Input: part model. Units: mm. Frame: model coordinates. A direction names the side the tool comes from. Round coordinates to 2 decimals unless told otherwise and drop trailing zeros. Write each loop counter-clockwise with the first axis right and the second up, starting at its lowest first coordinate (ties: lowest second). Pieces come first, ordered by that corner, then holes. Notation, with made-up numbers: (-13.5, -11) -> (-6.5, -11) arc R30 cw to (-6.5, 17) -> close; hole circle Ø10 at (-14.75, -40). An arc over 180 degrees is marked (long way). Write item = value, one per line.
```python
from build123d import *

# Parameters (mm, degrees)
EXTRUDE_1_DEPTH   = 15.1
SKETCH_2_R        = 2.5
EXTRUDE_2_DEPTH   = 1.5
EXTRUDE_3_DEPTH   = 1.5
M1_6X0_35_1_D     = 1.25
M1_6X0_35_1_DEPTH = 4.95
M1_6X0_35_1_TIP   = 0.375537887
EXTRUDE_4_DEPTH   = 14.9
SKETCH_7_3_W      = 1
SKETCH_7_3_H      = 2
EXTRUDE_5_DEPTH   = 12.9
SKETCH_8_R        = 2
EXTRUDE_6_DEPTH   = 1.1
EXTRUDE_7_DEPTH   = 1.5
SKETCH_10_R       = 1.2
SKETCH_10_R_2     = 0.65
EXTRUDE_13_DEPTH  = 25


with BuildPart() as part:
    # Sketch 1 → Extrude 1 (new body)
    with BuildSketch(Plane.XY):
        with BuildLine():
            Line((-40.194845485, 23.273623853), (-32.294845485, 23.273623853))
            ThreePointArc((-32.294845485, 23.273623853), (-30.880631923, 22.687837416), (-30.294845485, 21.273623853))
            Line((-30.294845485, 21.273623853), (-30.294845485, 11.373623853))
            ThreePointArc((-30.294845485, 11.373623853), (-30.880631923, 9.959410291), (-32.294845485, 9.373623853))
            Line((-32.294845485, 9.373623853), (-40.194845485, 9.373623853))
            ThreePointArc((-40.194845485, 9.373623853), (-41.609059048, 9.959410291), (-42.194845485, 11.373623853))
            Line((-42.194845485, 11.373623853), (-42.194845485, 21.273623853))
            ThreePointArc((-42.194845485, 21.273623853), (-41.609059048, 22.687837416), (-40.194845485, 23.273623853))
        make_face()
    extrude(amount=EXTRUDE_1_DEPTH)

    # Sketch 2 → Extrude 2 (add)
    with BuildSketch(Plane.XY.offset(15.1)):
        with Locations((-36.244845485, 16.323623853)):
            Circle(SKETCH_2_R)
    extrude(amount=EXTRUDE_2_DEPTH)

    # Sketch 3 → Extrude 3 (add)
    with BuildSketch(Plane(origin=(0, 23.273623853, 0), x_dir=(1, 0, 0), z_dir=(0, 1, 0))):
        with BuildLine():
            Line((-33.744845485, -10.6), (-38.744845485, -10.6))
            ThreePointArc((-38.744845485, -10.6), (-39.098398876, -10.746446609), (-39.244845485, -11.1))
            Line((-39.244845485, -11.1), (-39.244845485, -15.1))
            Line((-39.244845485, -15.1), (-38.744845485, -15.1))
            Line((-38.744845485, -15.1), (-38.744845485, -14.6))
            Line((-38.744845485, -14.6), (-38.744845485, -11.6))
            ThreePointArc((-38.744845485, -11.6), (-38.598398876, -11.246446609), (-38.244845485, -11.1))
            Line((-38.244845485, -11.1), (-34.244845485, -11.1))
            ThreePointArc((-34.244845485, -11.1), (-33.891292095, -11.246446609), (-33.744845485, -11.6))
            Line((-33.744845485, -11.6), (-33.744845485, -14.6))
            Line((-33.744845485, -14.6), (-33.744845485, -15.1))
            Line((-33.744845485, -15.1), (-33.244845485, -15.1))
            Line((-33.244845485, -15.1), (-33.244845485, -11.1))
            ThreePointArc((-33.244845485, -11.1), (-33.391292095, -10.746446609), (-33.744845485, -10.6))
        make_face()
    extrude(amount=EXTRUDE_3_DEPTH)

    # M1.6x0.35 _1
    with Locations(Plane(origin=(-32.294845485, 21.273623853, 15.1), x_dir=(1, 0, 0), z_dir=(0, 0, 1))):
        with Locations((0, 0), (-7.9, -9.9)):
            Hole(M1_6X0_35_1_D / 2, depth=M1_6X0_35_1_DEPTH)
            with Locations((0, 0, -(M1_6X0_35_1_DEPTH + M1_6X0_35_1_TIP / 2))):  # 118° drill point
                Cone(0, M1_6X0_35_1_D / 2, M1_6X0_35_1_TIP, mode=Mode.SUBTRACT)

    # Sketch 7 → Extrude 4 (add)
    with BuildSketch(Plane(origin=(0, 0, 0), x_dir=(-1, 0, 0), z_dir=(0, 0, -1))):
        with BuildLine():
            Line((36.244845485, 10.373623853), (36.244845485, 22.323623853))
            ThreePointArc((36.244845485, 22.323623853), (33.407571154, 21.610387927), (31.244845485, 19.640248644))
            Line((31.244845485, 19.640248644), (31.244845485, 17.373623853))
            Line((31.244845485, 17.373623853), (32.244845485, 17.373623853))
            Line((32.244845485, 17.373623853), (32.244845485, 15.373623853))
            Line((32.244845485, 15.373623853), (31.244845485, 15.373623853))
            Line((31.244845485, 15.373623853), (31.244845485, 13.006999063))
            ThreePointArc((31.244845485, 13.006999063), (33.072229159, 11.231030639), (35.471864244, 10.373623853))
            Line((35.471864244, 10.373623853), (36.244845485, 10.373623853))
        make_face()
        with BuildLine():
            ThreePointArc((41.244845485, 19.640248644), (39.082119816, 21.610387927), (36.244845485, 22.323623853))
            Line((36.244845485, 22.323623853), (36.244845485, 10.373623853))
            Line((36.244845485, 10.373623853), (37.017826727, 10.373623853))
            ThreePointArc((37.017826727, 10.373623853), (39.417461811, 11.231030639), (41.244845485, 13.006999063))
            Line((41.244845485, 13.006999063), (41.244845485, 15.373623853))
            Line((41.244845485, 15.373623853), (40.244845485, 15.373623853))
            Line((40.244845485, 15.373623853), (40.244845485, 17.373623853))
            Line((40.244845485, 17.373623853), (41.244845485, 17.373623853))
            Line((41.244845485, 17.373623853), (41.244845485, 19.640248644))
        make_face()
    extrude(amount=EXTRUDE_4_DEPTH)

    # Sketch 7_3 → Extrude 5 (add)
    with BuildSketch(Plane(origin=(0, 0, 0), x_dir=(-1, 0, 0), z_dir=(0, 0, -1))):
        Polygon((32.244845485, 17.373623853), (31.244845485, 17.373623853), (31.244845485, 16.373623853), (31.244845485, 15.373623853), (32.244845485, 15.373623853), align=None)
        with Locations((40.744845485, 16.373623853)):
            Rectangle(SKETCH_7_3_W, SKETCH_7_3_H)
    extrude(amount=EXTRUDE_5_DEPTH)

    # Sketch 8 → Extrude 6 (add)
    with BuildSketch(Plane(origin=(0, 0, -14.9), x_dir=(-1, 0, 0), z_dir=(0, 0, -1))):
        with Locations((36.244845485, 16.323623853)):
            Circle(SKETCH_8_R)
    extrude(amount=EXTRUDE_6_DEPTH)

    # Sketch 8_3 → Extrude 7 (add)
    with BuildSketch(Plane(origin=(0, 0, -14.9), x_dir=(-1, 0, 0), z_dir=(0, 0, -1))):
        Polygon((35.654303745, 20.200200691), (35.569268974, 20.376569105), (36.920421996, 21.028017883), (37.005456768, 20.851649469), align=None)
        Polygon((36.835387225, 12.447047016), (36.920421996, 12.270678601), (35.569268974, 11.619229823), (35.484234203, 11.795598237), align=None)
    extrude(amount=EXTRUDE_7_DEPTH)

    # Sketch 10 → Extrude 13 (add)
    # profile 1 of 2: a face of its own
    with BuildSketch(Plane(origin=(0, 23.273623853, 0), x_dir=(1, 0, 0), z_dir=(0, 1, 0))):
        with Locations(Location((-37.494845485, -13.35, 0), (0, 0, 90))):
            Circle(SKETCH_10_R)
        with Locations(Location((-37.494845485, -13.35, 0), (0, 0, 270))):
            Circle(SKETCH_10_R_2, mode=Mode.SUBTRACT)
    # profile 2 of 2: a face of its own
    with BuildSketch(Plane(origin=(0, 23.273623853, 0), x_dir=(1, 0, 0), z_dir=(0, 1, 0))):
        with Locations(Location((-34.994845485, -13.35, 0), (0, 0, 90))):
            Circle(SKETCH_10_R)
        with Locations(Location((-34.994845485, -13.35, 0), (0, 0, 270))):
            Circle(SKETCH_10_R_2, mode=Mode.SUBTRACT)
    extrude(amount=EXTRUDE_13_DEPTH)


solid = part.part
```
1) Cut plane B-B (z = 2). Return the cut outline in (x, y).
Solutions:
outline = (-42.19, 11.37) arc R2 ccw to (-40.19, 9.37) -> (-32.29, 9.37) arc R2 ccw to (-30.29, 11.37) -> (-30.29, 21.27) arc R2 ccw to (-32.29, 23.27) -> (-40.19, 23.27) arc R2 ccw to (-42.19, 21.27) -> close
2) First-contact query: P1, Ø1, axis at x = -32.29, y = 21.27, coming from the -Z side; P2, Ø1.6, axis at x = -36, y = 24, coming from the -Z side; P3, Ø1, axis at x = -35.5, y = 18.5, coming from the -Z side. Flat tips, straight axial feed; report the tip coordinate or a pass-through.
Solutions:
P1 = -14.9
P2 = 0
P3 = -16
3) Cut plane C-C (y = 34). Return the cut outline in (x, z), and give its area (3 significant figures).
Solutions:
outline = circle Ø2.4 at (-37.49, 13.35); circle Ø2.4 at (-34.99, 13.35); hole circle Ø1.3 at (-37.49, 13.35); hole circle Ø1.3 at (-34.99, 13.35)
area = 6.39 mm^2
4) Access query for faces 1 (the face through (-31.245, 16, -7)), 2 (the face through (-32.89, 21.46, 12.59)), 3 (the face through (-41, 15.374, -14)), 4 (the face through (-38.685, 35.599, 13.506)). Directions: +Z, -Z, +X, -X, +Y, -Y. A direction counts if a zero-diameter tool reaches every point of the face in a straight line with its end or side. Return the directions, or none.
Solutions:
face_1 = -Z, +X, +Y, -Y
face_2 = +Z
face_3 = -Z, -X
face_4 = +Y
5) Line query: L1, parallel to Z at x = -41, y = 15.5; L2, parallel to Y at x = -31.75, z = -14; L3, parallel to Z at x = -34.5, y = 37.5. Output: solid intervals per line, ascending. Write a range as from..to.
Solutions:
L1 = -12.9..15.1
L2 = 12.35..15.37, 17.37..20.3
L3 = 12.26..12.93, 13.77..14.44
6) Draft query along Z for faces 5 (the face through (-41, 16, -12.9)), 6 (the face through (-41.245, 16, -7)), 7 (the face through (-36.3, 23.274, 12.6)). Return one class per face: +Z half, -Z half, draft (parallel to the pull), parting line (faces both ways), or undercut.
Solutions:
face_5 = -Z half
face_6 = draft
face_7 = undercut
7) Cut plane A-A (z = 13.35). Count the separate pieces of the cut face and the enclosed holes in it, and give its area (3 significant figures).
Solutions:
separate_pieces = 1
enclosed_holes = 2
area = 216 mm^2
8) Cut plane D-D (z = -1.5). Return the cut outline in (x, y), and give its area (3 significant figures).
Solutions:
outline = (-41.24, 13.01) arc R6 ccw to (-37.02, 10.37) -> (-35.47, 10.37) arc R6 ccw to (-31.24, 13.01) -> (-31.24, 19.64) arc R6 ccw to (-41.24, 19.64) -> close
area = 104 mm^2
